Can you work these out from the model? Positions are in its coordinate system, mm. Face numbers are marked on the shaded views. A direction names the side the tool comes from. Give positions to 0.01 mm unless a question says otherwise; leave off trailing zeros. Order: outer loops, then holes, each group sorted by start corner. A loop starts at its lowest first (then second) coordinate and runs counter-clockwise, first axis right, second up. Notation, with made-up numbers: M -4.75,3 L 16.25,3 A27 cw 16.25,33 Z; hole C -3.75,44.5 d5. An arc over 180 degrees is marked long. Answer as a JSON object with one key per item and string values.
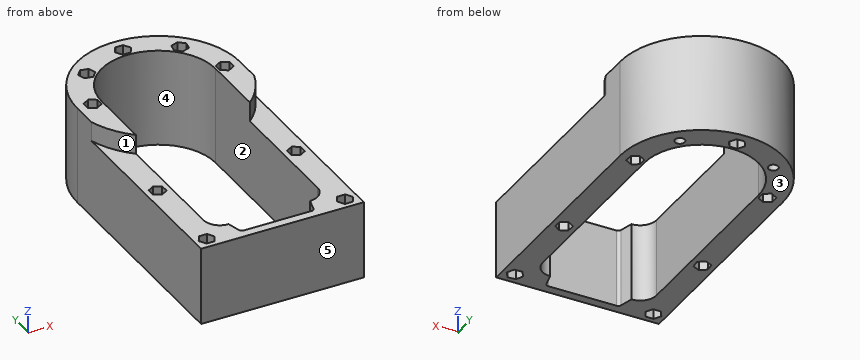
```python
from build123d import *

# Parameters (mm, degrees)
SALIENTE_EXTRUIR1_DEPTH = 60
CROQUIS2_R              = 3
CORTAR_EXTRUIR1_DEPTH   = 60
CORTAR_EXTRUIR2_DEPTH   = 6
CORTAR_EXTRUIR3_DEPTH   = 12
CROQUIS5_R              = 3
CORTAR_EXTRUIR4_DEPTH   = 48
CORTAR_EXTRUIR5_DEPTH   = 6
CORTAR_EXTRUIR6_DEPTH   = 6
CORTAR_EXTRUIR7_DEPTH   = 48


with BuildPart() as part:
    # Croquis1 → Saliente-Extruir1 (new body)
    with BuildSketch(Plane.XY):
        with BuildLine():
            Line((-50, 0), (-50, -141))
            Line((-50, -141), (50, -141))
            Line((50, -141), (50, 0))
            ThreePointArc((50, 0), (0, 50), (-50, 0))
        make_face()
        with BuildLine():
            Line((-35, 0), (-35, -116))
            ThreePointArc((-35, -116), (-32.071067812, -123.071067812), (-25, -126))
            Line((-25, -126), (25, -126))
            ThreePointArc((25, -126), (32.071067812, -123.071067812), (35, -116))
            Line((35, -116), (35, 0))
            ThreePointArc((35, 0), (0, 35), (-35, 0))
        make_face(mode=Mode.SUBTRACT)
    extrude(amount=SALIENTE_EXTRUIR1_DEPTH)

    # Croquis2 → Cortar-Extruir1 (cut)
    with BuildSketch(Plane.XY.offset(60)):
        with Locations((0, 40.605)):
            Circle(CROQUIS2_R)
        with Locations((28.71207085, 28.71207085)):
            Circle(CROQUIS2_R)
        with Locations((40.605, 0)):
            Circle(CROQUIS2_R)
        with Locations((-40.605, 0)):
            Circle(CROQUIS2_R)
        with Locations((-28.71207085, 28.71207085)):
            Circle(CROQUIS2_R)
    extrude(amount=-CORTAR_EXTRUIR1_DEPTH, mode=Mode.SUBTRACT)

    # Croquis3 → Cortar-Extruir2 (cut)
    with BuildSketch(Plane.XY.offset(60)):
        Polygon((4.907477288, 40.605), (2.453738644, 44.855), (-2.453738644, 44.855), (-4.907477288, 40.605), (-2.453738644, 36.355), (2.453738644, 36.355), align=None)
        Polygon((33.365133185, 30.271668311), (29.687950997, 33.521539768), (25.034888662, 31.961942307), (24.059008515, 27.152473389), (27.736190704, 23.902601932), (32.389253039, 25.462199393), align=None)
        Polygon((40.605, -4.907477288), (44.855, -2.453738644), (44.855, 2.453738644), (40.605, 4.907477288), (36.355, 2.453738644), (36.355, -2.453738644), align=None)
        Polygon((-33.528922476, 29.650832668), (-31.933488245, 25.009935885), (-27.11663662, 24.071174067), (-23.895219225, 27.773309032), (-25.490653455, 32.414205815), (-30.30750508, 33.352967633), align=None)
        Polygon((-40.605, 4.907477288), (-44.855, 2.453738644), (-44.855, -2.453738644), (-40.605, -4.907477288), (-36.355, -2.453738644), (-36.355, 2.453738644), align=None)
    extrude(amount=-CORTAR_EXTRUIR2_DEPTH, mode=Mode.SUBTRACT)

    # Croquis4 → Cortar-Extruir3 (cut)
    with BuildSketch(Plane.XY.offset(60)):
        with BuildLine():
            Line((-50, -16.007810594), (-50, -141))
            Line((-50, -141), (50, -141))
            Line((50, -141), (50, -16.007810594))
            ThreePointArc((50, -16.007810594), (0, -52.5), (-50, -16.007810594))
        make_face()
    extrude(amount=-CORTAR_EXTRUIR3_DEPTH, mode=Mode.SUBTRACT)

    # Croquis5 → Cortar-Extruir4 (cut)
    with BuildSketch(Plane.XY.offset(48)):
        with Locations((-42.5, -77.565594803)):
            Circle(CROQUIS5_R)
        with Locations((-42.5, -133.5)):
            Circle(CROQUIS5_R)
        with Locations((42.5, -77.565594803)):
            Circle(CROQUIS5_R)
        with Locations((42.5, -133.5)):
            Circle(CROQUIS5_R)
    extrude(amount=-CORTAR_EXTRUIR4_DEPTH, mode=Mode.SUBTRACT)

    # Croquis6 → Cortar-Extruir5 (cut)
    with BuildSketch(Plane.XY.offset(48)):
        Polygon((-42.421317924, -82.472441292), (-38.21120525, -79.950877371), (-38.289887326, -75.044030882), (-42.578682076, -72.658748314), (-46.78879475, -75.180312235), (-46.710112674, -80.087158724), align=None)
        Polygon((42.5, -82.473072091), (46.75, -80.019333447), (46.75, -75.111856159), (42.5, -72.658117515), (38.25, -75.111856159), (38.25, -80.019333447), align=None)
        Polygon((-40.063566251, -129.240055878), (-44.971002953, -129.260014418), (-47.407436703, -133.519958539), (-44.936433749, -137.759944122), (-40.028997047, -137.739985582), (-37.592563297, -133.480041461), align=None)
        Polygon((44.895973885, -129.217168871), (39.988946385, -129.283610185), (37.5929725, -133.566441313), (40.104026115, -137.782831129), (45.011053615, -137.716389815), (47.4070275, -133.433558687), align=None)
    extrude(amount=-CORTAR_EXTRUIR5_DEPTH, mode=Mode.SUBTRACT)

    # Croquis7 → Cortar-Extruir6 (cut)
    with BuildSketch(Plane(origin=(0, 0, 0), x_dir=(-1, 0, 0), z_dir=(0, 0, -1))):
        Polygon((2.357863822, 44.908929778), (-2.548380612, 44.798934857), (-4.906244434, 40.49500508), (-2.357863822, 36.301070222), (2.548380612, 36.411065143), (4.906244434, 40.71499492), align=None)
        Polygon((-40.614441302, 4.907468206), (-44.859712786, 2.445557696), (-44.850271484, -2.461910511), (-40.595558698, -4.907468206), (-36.350287214, -2.445557696), (-36.359728516, 2.461910511), align=None)
        Polygon((44.882492584, -2.405491744), (44.826963251, 2.50167137), (40.549470667, 4.907163114), (36.327507416, 2.405491744), (36.383036749, -2.50167137), (40.660529333, -4.907163114), align=None)
        Polygon((-42.131373877, -72.671981811), (-46.553680106, -74.79954872), (-46.922306229, -79.693161712), (-42.868626123, -82.459207795), (-38.446319894, -80.331640886), (-38.077693771, -75.438027894), align=None)
        Polygon((42.084370643, -72.675749655), (38.057455203, -75.480617811), (38.47308456, -80.370462959), (42.915629357, -82.455439951), (46.942544797, -79.650571795), (46.52691544, -74.760726647), align=None)
        Polygon((47.407477288, -133.5), (44.953738644, -129.25), (40.046261356, -129.25), (37.592522712, -133.5), (40.046261356, -137.75), (44.953738644, -137.75), align=None)
        Polygon((-44.636850652, -137.917827818), (-39.742474206, -137.559480857), (-37.605623555, -133.14165304), (-40.363149348, -129.082172182), (-45.257525794, -129.440519143), (-47.394376445, -133.85834696), align=None)
    extrude(amount=-CORTAR_EXTRUIR6_DEPTH, mode=Mode.SUBTRACT)

    # Croquis8 → Cortar-Extruir7 (cut)
    with BuildSketch(Plane.XY.offset(48)):
        with BuildLine():
            Line((-22.892371948, -134.008986599), (-25, -126))
            Line((-25, -126), (25, -126))
            Line((25, -126), (22.892371948, -134.008986599))
            ThreePointArc((22.892371948, -134.008986599), (22.17929347, -135.083978093), (20.958222873, -135.5))
            Line((20.958222873, -135.5), (-20.958222873, -135.5))
            ThreePointArc((-20.958222873, -135.5), (-22.17929347, -135.083978093), (-22.892371948, -134.008986599))
        make_face()
    extrude(amount=-CORTAR_EXTRUIR7_DEPTH, mode=Mode.SUBTRACT)


solid = part.part
```
1) I want a section at C-C on y = -23. Write out the boundary of the cut face in (x, z), and give its area (3 significant figures).
Results found:
{"outline": "M -50,0 L -35,0 L -35,60 L -47.19,60 L -47.19,48 L -50,48 Z; M 35,0 L 50,0 L 50,48 L 47.19,48 L 47.19,60 L 35,60 Z", "area": "1,730 mm²"}
2) For the marked faces 4 and 5, which set-ups out of +Z, -Z, +X, -X, +Y, -Y let a thin tool reach every point of the face, with its end or its side?
Results found:
{"face 4": "+Z, -Z", "face 5": "+Z, -Z, +X, -X, -Y"}
3) I want a section at B-B on x = 0. Write out the boundary of the cut face in (y, z) (3 decimals), and give its area (3 significant figures).
Results found:
{"outline": "M -141,0 L -135.5,0 L -135.5,48 L -141,48 Z; M 35,0 L 36.354,0 L 36.354,6 L 37.605,6 L 37.605,54 L 36.355,54 L 36.355,60 L 35,60 Z; M 43.605,6 L 44.856,6 L 44.856,0 L 50,0 L 50,60 L 44.855,60 L 44.855,54 L 43.605,54 Z", "area": "774 mm²"}
4) I want a section at A-A on y = -65.5. Write out the boundary of the cut face in (x, z), and give its area (3 significant figures).
Results found:
{"outline": "M -50,0 L -35,0 L -35,48 L -50,48 Z; M 35,0 L 50,0 L 50,48 L 35,48 Z", "area": "1,440 mm²"}
5) I'm going to push flat-ended pins straight in: pin 1 Ø3 at (x, z) = (9.5, 32) entering from +Y; pin 2 Ø8 at (x, y) = (40.605, 0) entering from -Z; pin 3 Ø10 at (x, y) = (27.5, 28.5) entering from +Z; pin 4 Ø1 at (x, z) = (4.5, 19) entering from +Y. Where does each tip first touch, or does it pass through?
Results found:
{"pin 1": "stops at y = 49.36", "pin 2": "stops at z = 6", "pin 3": "stops at z = 60", "pin 4": "stops at y = 49.84"}
6) Thinking about a two-plate mould opening in X: for the marked faces 1, 2 and 3, which applies, pulls with the +X half, pulls with the -X half, needs draft (parallel to the pull), parting line crosses it, or undercut?
Results found:
{"face 1": "pulls with the -X half", "face 2": "undercut", "face 3": "needs draft"}
7) I need wall thicknesses on L1, parallel to Y at x = 0, z = 33 (3 decimals); L2, parallel to Y at x = -42, z = 18; L3, parallel to X at y = -1, z = 44.5. Which ranges of each line are inside material? Lowest first, please.
Results found:
{"L1": "y = -141 to -135.5, 35 to 37.605, 43.605 to 50", "L2": "y = -141 to -136.46, -130.54 to -80.52, -74.61 to -2.66, 2.66 to 27.13", "L3": "x = -50 to -43.43, -37.78 to -35, 35 to 37.78, 43.43 to 50"}
